Source: CAD feature listing. Evaluate the final solid. Frame: model axes, mm. Face numbers are marked on the shaded views. Give positions to 0.01 mm unless a question says otherwise; leave off trailing zeros. Order: outer loops, then holes, each group sorted by start corner. A loop starts at its lowest first (then second) coordinate and runs counter-clockwise, first axis right, second up.
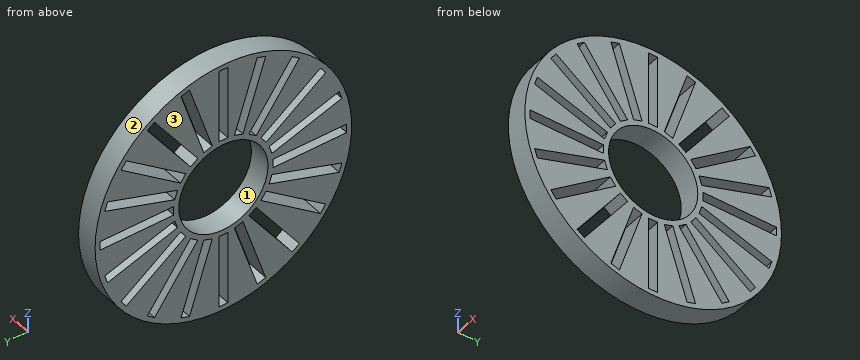
Autodesk Inventor part; units mm, degrees
ref_plane "YZ Plane" through (0, 0, 0) normal (1, 0, 0) x (0, 1, 0)
ref_plane "XZ Plane" through (0, 0, 0) normal (0, 1, 0) x (-1, 0, 0)
ref_plane "XY Plane" through (0, 0, 0) normal (0, 0, 1) x (1, 0, 0)
sketch "Sketch1" plane through (0, 0, 0) normal (1, 0, 0) x (0, 1, 0)
  circle A0 centre (0, 0) radius 4
  circle A1 centre (0, 0) radius 11.5
  dimension "d0" = 8
  dimension "d1" = 23
extrude "Extrusion1" add sketch "Sketch1" along normal mid plane 2
sketch "Sketch4" plane through (1, 0, 0) normal (1, 0, 0) x (0, 0, -1)
  circle A0 centre (0, 0) radius 11.5 construction
  circle A1 centre (0, 0) radius 4 construction
  line L0 (-11.5, 0) -> (-4, 0) construction
  line L1 (-11.05, -0.4) -> (-4.45, -0.4)
  line L2 (-4.45, -0.4) -> (-4.45, 0.4)
  line L3 (-4.45, 0.4) -> (-11.05, 0.4)
  line L4 (-11.05, 0.4) -> (-11.05, -0.4)
  line L5 (-11.05, -0.4) -> (-4.45, 0.4) construction
  line L6 (-4.45, -0.4) -> (-11.05, 0.4) construction
  line L7 (-4.3558, -0.9947) -> (-10.6328, -3.0342)
  line L8 (-4.1086, -1.7555) -> (-4.3558, -0.9947)
  line L9 (-10.3856, -3.7951) -> (-4.1086, -1.7555)
  line L10 (-10.6328, -3.0342) -> (-10.3856, -3.7951)
  line L11 (-3.8352, -2.292) -> (-9.1748, -6.1714)
  line L12 (-3.365, -2.9393) -> (-3.8352, -2.292)
  line L13 (-8.7045, -6.8186) -> (-3.365, -2.9393)
  line L14 (-9.1748, -6.1714) -> (-8.7045, -6.8186)
  line L15 (-2.9393, -3.365) -> (-6.8186, -8.7045)
  line L16 (-2.292, -3.8352) -> (-2.9393, -3.365)
  line L17 (-6.1714, -9.1748) -> (-2.292, -3.8352)
  line L18 (-6.8186, -8.7045) -> (-6.1714, -9.1748)
  line L19 (-1.7555, -4.1086) -> (-3.7951, -10.3856)
  line L20 (-0.9947, -4.3558) -> (-1.7555, -4.1086)
  line L21 (-3.0342, -10.6328) -> (-0.9947, -4.3558)
  line L22 (-3.7951, -10.3856) -> (-3.0342, -10.6328)
  line L23 (-0.4, -4.45) -> (-0.4, -11.05)
  line L24 (0.4, -4.45) -> (-0.4, -4.45)
  line L25 (0.4, -11.05) -> (0.4, -4.45)
  line L26 (-0.4, -11.05) -> (0.4, -11.05)
  line L27 (0.9947, -4.3558) -> (3.0342, -10.6328)
  line L28 (1.7555, -4.1086) -> (0.9947, -4.3558)
  line L29 (3.7951, -10.3856) -> (1.7555, -4.1086)
  line L30 (3.0342, -10.6328) -> (3.7951, -10.3856)
  line L31 (2.292, -3.8352) -> (6.1714, -9.1748)
  line L32 (2.9393, -3.365) -> (2.292, -3.8352)
  line L33 (6.8186, -8.7045) -> (2.9393, -3.365)
  line L34 (6.1714, -9.1748) -> (6.8186, -8.7045)
  line L35 (3.365, -2.9393) -> (8.7045, -6.8186)
  line L36 (3.8352, -2.292) -> (3.365, -2.9393)
  line L37 (9.1748, -6.1714) -> (3.8352, -2.292)
  line L38 (8.7045, -6.8186) -> (9.1748, -6.1714)
  line L39 (4.1086, -1.7555) -> (10.3856, -3.7951)
  line L40 (4.3558, -0.9947) -> (4.1086, -1.7555)
  line L41 (10.6328, -3.0342) -> (4.3558, -0.9947)
  line L42 (10.3856, -3.7951) -> (10.6328, -3.0342)
  line L43 (4.45, -0.4) -> (11.05, -0.4)
  line L44 (4.45, 0.4) -> (4.45, -0.4)
  line L45 (11.05, 0.4) -> (4.45, 0.4)
  line L46 (11.05, -0.4) -> (11.05, 0.4)
  line L47 (4.3558, 0.9947) -> (10.6328, 3.0342)
  line L48 (4.1086, 1.7555) -> (4.3558, 0.9947)
  line L49 (10.3856, 3.7951) -> (4.1086, 1.7555)
  line L50 (10.6328, 3.0342) -> (10.3856, 3.7951)
  line L51 (3.8352, 2.292) -> (9.1748, 6.1714)
  line L52 (3.365, 2.9393) -> (3.8352, 2.292)
  line L53 (8.7045, 6.8186) -> (3.365, 2.9393)
  line L54 (9.1748, 6.1714) -> (8.7045, 6.8186)
  line L55 (2.9393, 3.365) -> (6.8186, 8.7045)
  line L56 (2.292, 3.8352) -> (2.9393, 3.365)
  line L57 (6.1714, 9.1748) -> (2.292, 3.8352)
  line L58 (6.8186, 8.7045) -> (6.1714, 9.1748)
  line L59 (1.7555, 4.1086) -> (3.7951, 10.3856)
  line L60 (0.9947, 4.3558) -> (1.7555, 4.1086)
  line L61 (3.0342, 10.6328) -> (0.9947, 4.3558)
  line L62 (3.7951, 10.3856) -> (3.0342, 10.6328)
  line L63 (0.4, 4.45) -> (0.4, 11.05)
  line L64 (-0.4, 4.45) -> (0.4, 4.45)
  line L65 (-0.4, 11.05) -> (-0.4, 4.45)
  line L66 (0.4, 11.05) -> (-0.4, 11.05)
  line L67 (-0.9947, 4.3558) -> (-3.0342, 10.6328)
  line L68 (-1.7555, 4.1086) -> (-0.9947, 4.3558)
  line L69 (-3.7951, 10.3856) -> (-1.7555, 4.1086)
  line L70 (-3.0342, 10.6328) -> (-3.7951, 10.3856)
  line L71 (-2.292, 3.8352) -> (-6.1714, 9.1748)
  line L72 (-2.9393, 3.365) -> (-2.292, 3.8352)
  line L73 (-6.8186, 8.7045) -> (-2.9393, 3.365)
  line L74 (-6.1714, 9.1748) -> (-6.8186, 8.7045)
  line L75 (-3.365, 2.9393) -> (-8.7045, 6.8186)
  line L76 (-3.8352, 2.292) -> (-3.365, 2.9393)
  line L77 (-9.1748, 6.1714) -> (-3.8352, 2.292)
  line L78 (-8.7045, 6.8186) -> (-9.1748, 6.1714)
  line L79 (-4.1086, 1.7555) -> (-10.3856, 3.7951)
  line L80 (-4.3558, 0.9947) -> (-4.1086, 1.7555)
  line L81 (-10.6328, 3.0342) -> (-4.3558, 0.9947)
  line L82 (-10.3856, 3.7951) -> (-10.6328, 3.0342)
  point P0 (-7.75, 0)
  dimension "d15" = 6.6
  dimension "d16" = 0.8
  dimension "d19" = 360
extrude "Extrusion4" cut sketch "Sketch4" against normal blind 5
properties part number "encoder"
(1) Section C-C, the plane x = 0.35. Count the separate pieces of the cut face and the enclosed holes in it, plus the area to 3 significant figures.
(2) Draft query along Z for the marked faces 1, 2 and 3. Return one class per face: +Z half, -Z half, draft (parallel to the pull), parting line (faces both ways), or undercut.
(3) Section A-A, the plane y = 0. Return loops of the section in (x, z).
(4) Line query: line 1 along Z through (x, y) = (-0.55, 0); line 2 along Z through (x, y) = (-0.55, -9.5); line 3 along Z through (x, y) = (-0.8, -7.5). Output: solid intervals per line, ascending.
(5) Pin query (flat end, axial travel): pin 1 Ø7 at (y, z) = (0, 0) entering from -X; pin 2 Ø0.6 at (x, z) = (0, -8.5) entering from -Y. Return the tip coordinate at first contact, or that it passes through.
Checks:
1. separate pieces: 1
1. enclosed holes: 21
1. area: 260 mm2
2. face 1: undercut
2. face 2: parting line
2. face 3: draft
3. outline: (-1, -11.5) - (1, -11.5) - (1, -11.05) - (-1, -11.05) - close; (-1, -4.45) - (1, -4.45) - (1, -4) - (-1, -4) - close; (-1, 4) - (1, 4) - (1, 4.45) - (-1, 4.45) - close; (-1, 11.05) - (1, 11.05) - (1, 11.5) - (-1, 11.5) - close
4. line 1: z = -11.5 to -11.05, -4.45 to -4, 4 to 4.45, 11.05 to 11.5
4. line 2: z = -6.48 to -3.51, -2.67 to -0.4, 0.4 to 2.67, 3.51 to 6.48
4. line 3: z = -8.72 to -5.94, -4.95 to -2.86, -2.02 to -0.4, 0.4 to 2.02, 2.86 to 4.95, 5.94 to 8.72
5. pin 1: passes through
5. pin 2: stops at y = -8.06
